Source: CAD feature listing. Evaluate the final solid. Frame: model axes, mm. Give positions to 0.01 mm unless a question says otherwise; leave off trailing zeros. Loops run counter-clockwise (first coordinate to the right, second up) from the corner with the lowest first, then second, coordinate; pieces in that order, holes last. Notation, with made-up numbers: M -31,66 L -21,66 A31 ccw -21,94 Z; hole C 29.5,82 d9. An arc over 180 degrees is marked long. Write item = value, one per line.
from build123d import *

# Parameters (mm, degrees)
BASE_FLANGE1_DEPTH = 30
M3_TAPPED_HOLE1_D  = 2.5
M3_TAPPED_HOLE2_D  = 2.5


# Sheet-metal steps are written as plain solids
with BuildPart() as part:
    # Sketch1 → Base-Flange1 (new, symmetric)
    with BuildSketch(Plane.XY):
        with BuildLine():
            Line((10, 0), (3.5, 0))
            ThreePointArc((3.5, 0), (1.025126266, 1.025126266), (0, 3.5))
            Line((0, 3.5), (0, 10))
            Line((0, 10), (2, 10))
            Line((2, 10), (2, 3.5))
            ThreePointArc((2, 3.5), (2.439339828, 2.439339828), (3.5, 2))
            Line((3.5, 2), (10, 2))
            Line((10, 2), (10, 0))
        make_face()
    extrude(amount=BASE_FLANGE1_DEPTH, both=True)

    # M3 Tapped Hole1 (through all)
    with Locations(Plane(origin=(2, 0, 0), x_dir=(0, 0, -1), z_dir=(1, 0, 0))):
        with Locations((-26, 6), (26, 6)):
            Hole(M3_TAPPED_HOLE1_D / 2)

    # M3 Tapped Hole2 (through all)
    with Locations(Plane(origin=(0, 2, 0), x_dir=(1, 0, 0), z_dir=(0, 1, 0))):
        with Locations((6, -26), (6, 26)):
            Hole(M3_TAPPED_HOLE2_D / 2)


solid = part.part
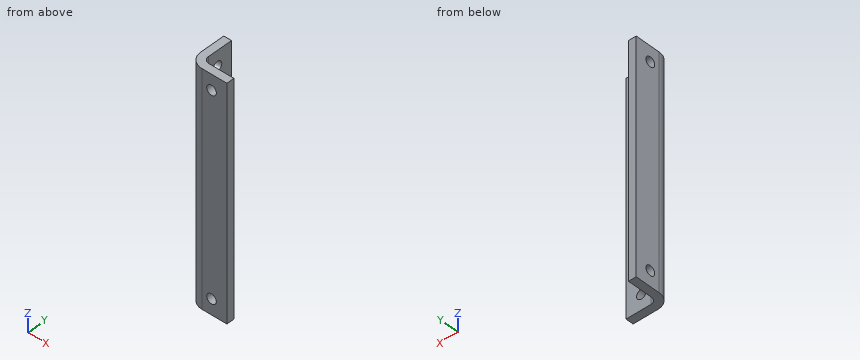
1. First-contact query: pin 1 Ø2 at (y, z) = (5.5, 3) entering from +X; pin 2 Ø5 at (x, z) = (7.5, -10) entering from +Y; pin 3 Ø1.5 at (y, z) = (6, 26) entering from +X. Flat tips, straight axial feed; report the tip coordinate or a pass-through.
Derived:
pin_1 = 2
pin_2 = 2
pin_3 = through
2. Cut plane D-D, the plane z = 8. Return the cut outline in (x, y).
Derived:
outline = M 0,3.5 A3.5 ccw 3.5,0 L 10,0 L 10,2 L 3.5,2 A1.5 cw 2,3.5 L 2,10 L 0,10 Z
3. Cut plane B-B, the plane y = 6. Return the cut outline in (x, z), then the cut area to 3 significant figures.
Derived:
outline = M 0,-30 L 2,-30 L 2,-27.25 L 0,-27.25 Z; M 0,-24.75 L 2,-24.75 L 2,24.75 L 0,24.75 Z; M 0,27.25 L 2,27.25 L 2,30 L 0,30 Z
area = 110 mm²
4. Cut plane A-A, the plane z = 26. Return the cut outline in (x, y).
Derived:
outline = M 0,3.5 A3.5 ccw 3.5,0 L 4.75,0 L 4.75,2 L 3.5,2 A1.5 cw 2,3.5 L 2,4.75 L 0,4.75 Z; M 0,7.25 L 2,7.25 L 2,10 L 0,10 Z; M 7.25,0 L 10,0 L 10,2 L 7.25,2 Z
5. Material intervals for probe 1 along Z at (x, y) = (6, 1.05); probe 2 along Y at (x, z) = (5, -17), sorted ascending. Write a range as from..to.
Derived:
probe_1 = -30..-27.25, -24.75..24.75, 27.25..30
probe_2 = 0..2
